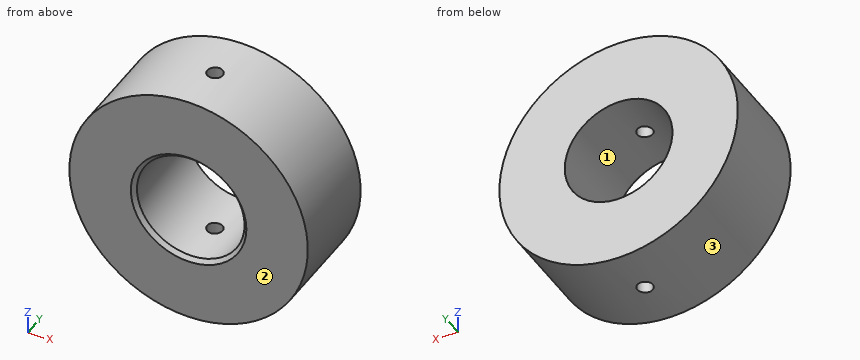
```python
from build123d import *

# Parameters (mm, degrees)
SKETCH1_R                        = 31
BOSS_EXTRUDE1_DEPTH              = 12.5
CUT_EXTRUDE1_DEPTH               = 46.587827323
CUT_EXTRUDE1_DEPTH_BACK          = 46.587827323
SKETCH2_R                        = 2
M30X2_0_TAPPED_HOLE1_D           = 28
M30X2_0_TAPPED_HOLE1_DEPTH       = 25
M30X2_0_TAPPED_HOLE1_CSINK_D     = 30.05
M30X2_0_TAPPED_HOLE1_CSINK_ANGLE = 90
M30X2_0_TAPPED_HOLE1_TIP         = 8.412048666


with BuildPart() as part:
    # Sketch1 → Boss-Extrude1 (new, symmetric)
    with BuildSketch(Plane(origin=(0, 0, 0), x_dir=(1, 0, 0), z_dir=(0, 1, 0))):
        with Locations(Location((0, 0, 0), (0, 0, 270))):
            Circle(SKETCH1_R)
    extrude(amount=BOSS_EXTRUDE1_DEPTH, both=True)

    # Sketch2 → Cut-Extrude1 (cut, two sides: drawn at the far end of the back side and taken through both)
    with BuildSketch(Plane.XY.offset(-CUT_EXTRUDE1_DEPTH_BACK)):
        Circle(SKETCH2_R)
    extrude(amount=CUT_EXTRUDE1_DEPTH + CUT_EXTRUDE1_DEPTH_BACK, mode=Mode.SUBTRACT)

    # M30x2.0 Tapped Hole1
    with Locations(Plane(origin=(0, -12.5, 0), x_dir=(-1, 0, 0), z_dir=(0, -1, 0))):
        with Locations((0, 0)):
            CounterSinkHole(M30X2_0_TAPPED_HOLE1_D / 2, M30X2_0_TAPPED_HOLE1_CSINK_D / 2, depth=M30X2_0_TAPPED_HOLE1_DEPTH, counter_sink_angle=M30X2_0_TAPPED_HOLE1_CSINK_ANGLE)
            with Locations((0, 0, -(M30X2_0_TAPPED_HOLE1_DEPTH + M30X2_0_TAPPED_HOLE1_TIP / 2))):  # 118° drill point
                Cone(0, M30X2_0_TAPPED_HOLE1_D / 2, M30X2_0_TAPPED_HOLE1_TIP, mode=Mode.SUBTRACT)


solid = part.part
```
Can you work these out from the model? Positions are in its coordinate system, mm. Face numbers are marked on the shaded views. Round coordinates to 2 decimals unless told otherwise and drop trailing zeros. Loops run counter-clockwise (first coordinate to the right, second up) from the corner with the lowest first, then second, coordinate; pieces in that order, holes last.
Item 1: Will these pins go through, and if not, where does the flat tip stop? pin 1 Ø3 at (y, z) = (0, -3.5) entering from +X; pin 2 Ø4 at (y, z) = (-0.5, -23) entering from -X; pin 3 Ø4 at (x, y) = (-13, -0.5) entering from +Z; pin 4 Ø3 at (x, y) = (0, 0) entering from -Z.
Item 2: Suppose I cut it at D-D, the plane y = 0. Write out the boundary of the cut face in (x, z).
Item 3: Suppose I cut it at A-A, the plane z = 0. Write out the boundary of the cut face in (x, y) (3 decimals), then the cut area to 3 significant figures.
Item 4: If we mould it in two halves opening along X, with no side actions, what happens to the marked faces 1, 2 and 3? For each: +X half, -X half, draft (parallel to the pull), parting line (faces both ways), or undercut.
Item 5: Suppose I cut it at B-B, the plane x = 0. Write out the boundary of the cut face in (y, z) (3 decimals), then the cut area to 3 significant figures.
Item 6: Please list where these lines run through material, in increasing order: L1, parallel to Y at x = 0, z = 20; L2, parallel to Z at x = 0, y = -2.5; L3, parallel to Z at x = -12.5, y = -11.
Item 7: Suppose I cut it at C-C, the plane y = 7.25. Write out the boundary of the cut face in (x, z), then the cut area to 3 significant figures.
Reported:
1. pin 1: stops at x = 30.94
1. pin 2: stops at x = -22.8
1. pin 3: stops at z = 28.98
1. pin 4: passes through
2. outline: (-2, -30.94) - (-2, -13.86) arc R14 cw to (-2, 13.86) - (-2, 30.94) arc R31 ccw to start; (2, -30.94) arc R31 ccw to (2, 30.94) - (2, 13.86) arc R14 cw to (2, -13.86) - close
3. outline: (-31, -12.5) - (-15.025, -12.5) - (-14, -11.475) - (-14, 12.5) - (-31, 12.5) - close; (14, -11.475) - (15.025, -12.5) - (31, -12.5) - (31, 12.5) - (14, 12.5) - close
3. area: 849 mm2
4. face 1: undercut
4. face 2: draft
4. face 3: parting line
5. outline: (-12.5, -31) - (-2, -31) - (-2, -14) - (-11.475, -14) - (-12.5, -15.025) - close; (-12.5, 15.025) - (-11.475, 14) - (-2, 14) - (-2, 31) - (-12.5, 31) - close; (2, -31) - (12.5, -31) - (12.5, -14) - (2, -14) - close; (2, 14) - (12.5, 14) - (12.5, 31) - (2, 31) - close
5. area: 713 mm2
6. L1: y = -12.5 to -2, 2 to 12.5
6. L2: z = -31 to -14, 14 to 31
6. L3: z = -28.37 to -6.3, 6.3 to 28.37
7. outline: circle Ø62 at (0, 0); hole circle Ø28 at (0, 0)
7. area: 2,400 mm2
